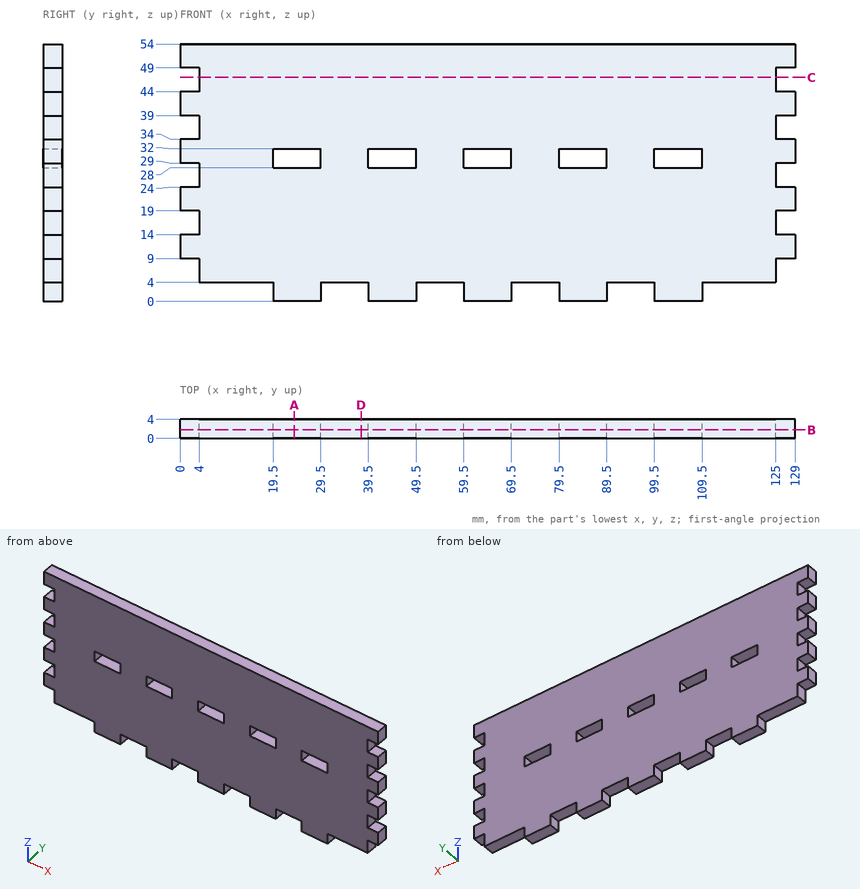
Check sheet for the drawn part. Datum: minimum x, y, z corner. Units: mm. Give positions to 0.01 mm unless a question says otherwise; leave off trailing zeros. Loops run counter-clockwise (first coordinate to the right, second up) from the corner with the lowest first, then second, coordinate; pieces in that order, holes last. Notation, with made-up numbers: M 54.5,33 L 91.5,33 A28 cw 91.5,72 Z; hole C 39,76 d1. An arc over 180 degrees is marked long. Return JSON: item names as keys, results as strings.
1) Gauge pin test, flat ends, axial feed: P1, Ø2, axis at x = 54, y = 2, coming from the -Z side; P2, Ø2, axis at y = 2.5, z = 2.5, coming from the -X side; P3, Ø1.2, axis at y = 2, z = 36.5, coming from the -X side. Record the tip position at first contact, or that the pin passes through.
Findings:
{"P1": "stops at z = 4", "P2": "stops at x = 19.5", "P3": "stops at x = 4"}
2) Section check B-B, the plane y = 1.8. Count the separate pieces of the cut face and the enclosed holes in it, and give its area (3 significant figures).
Findings:
{"separate pieces": "1", "enclosed holes": "5", "area": "6,250 mm2"}
3) Material ranges on L1, parallel to Z at x = 103.5, y = 0.75; L2, parallel to X at y = 1.55, z = 36; L3, parallel to Z at x = 97, y = 1.05, recorded low to high. Write a range as [from, to].
Findings:
{"L1": "z = [0, 28], [32, 54]", "L2": "x = [4, 125]", "L3": "z = [4, 54]"}
4) Section check C-C, the plane z = 47. Enter the section's corners in (x, y), and give its area (3 significant figures).
Findings:
{"outline": "M 4,0 L 125,0 L 125,4 L 4,4 Z", "area": "484 mm2"}
5) Section check A-A, the plane x = 24. Enter the section's corners in (y, z).
Findings:
{"outline": "M 0,0 L 4,0 L 4,28 L 0,28 Z; M 0,32 L 4,32 L 4,54 L 0,54 Z"}
6) Section check D-D, the plane x = 38. Enter the section's corners in (y, z), and give its area (3 significant figures).
Findings:
{"outline": "M 0,4 L 4,4 L 4,54 L 0,54 Z", "area": "200 mm2"}
